Design review of the part built by this model. Coordinates are the model's own, in mm. Face numbers are marked on the shaded views. Give positions to 0.01 mm unless a question says otherwise; leave off trailing zeros. Order: outer loops, then holes, each group sorted by start corner. A loop starts at its lowest first (then second) coordinate and runs counter-clockwise, first axis right, second up.
```python
from build123d import *

# Parameters (mm, degrees)
F0_W        = 40
F0_H        = 30
F0_R        = 2.6
F1_DEPTH    = 6
F2_T1_DEPTH = 31


# Not quite as in the source:
# - a fillet or chamfer that OpenCascade refuses, or shapes differently, is made with other operations: its cross-section is extruded or revolved along the edge and cut away or added


with BuildPart() as f1:
    # F0 (on Top) → F1 (new body)
    with BuildSketch(Plane.XY):
        Rectangle(F0_W, F0_H)
        with Locations((-10, -7)):
            Circle(F0_R, mode=Mode.SUBTRACT)
        with Locations((10, 0)):
            Circle(F0_R, mode=Mode.SUBTRACT)
    extrude(amount=F1_DEPTH)

    # F2: fillet of radius 5 on 4 edges, made by hand

    # F2_s2 → F2_t1 (cut)
    with BuildSketch(Plane.XY.offset(-12.5)):
        with BuildLine():
            add(Edge.make_bspline(
                [(-20, -10), (-20, -15), (-15, -15)],
                knots=[0, 0, 0, 1, 1, 1], degree=2, weights=[1, 1, 1]))
            Line((-15, -15), (-20, -15))
            Line((-20, -15), (-20, -10))
        make_face()
        with BuildLine():
            add(Edge.make_bspline(
                [(15, -15), (20, -15), (20, -10)],
                knots=[0, 0, 0, 1, 1, 1], degree=2, weights=[1, 1, 1]))
            Line((20, -10), (20, -15))
            Line((20, -15), (15, -15))
        make_face()
        with BuildLine():
            add(Edge.make_bspline(
                [(15, 15), (20, 15), (20, 10)],
                knots=[0, 0, 0, 1, 1, 1], degree=2, weights=[1, 1, 1]))
            Line((20, 10), (20, 15))
            Line((20, 15), (15, 15))
        make_face()
        with BuildLine():
            add(Edge.make_bspline(
                [(-15, 15), (-20, 15), (-20, 10)],
                knots=[0, 0, 0, 1, 1, 1], degree=2, weights=[1, 1, 1]))
            Line((-20, 10), (-20, 15))
            Line((-20, 15), (-15, 15))
        make_face()
    extrude(amount=F2_T1_DEPTH, mode=Mode.SUBTRACT)


solid = f1.part
```
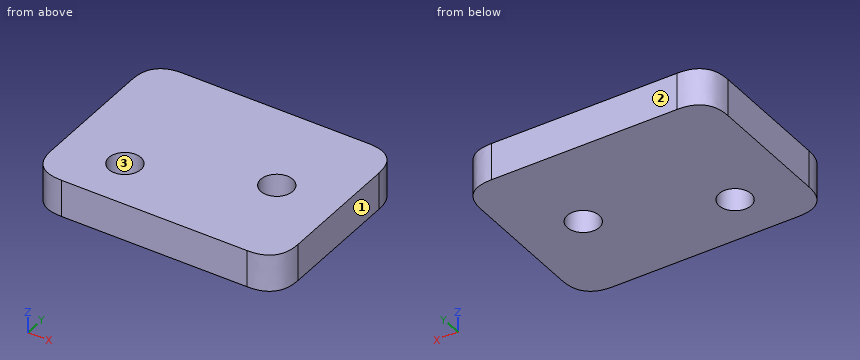
1. Take a section at B-B (y = 0). State the section outline as (x, z) points.
Recorded:
outline: (-20, 0) - (7.4, 0) - (7.4, 6) - (-20, 6) - close; (12.6, 0) - (20, 0) - (20, 6) - (12.6, 6) - close
2. Take a section at C-C (z = 1.75). State how many separate pieces and enclosed holes the cut face has, then the cut area to 3 significant figures.
Recorded:
separate pieces: 1
enclosed holes: 2
area: 1,140 mm2
3. Take a section at A-A (x = -11). State the section outline as (y, z) points.
Recorded:
outline: (-15, 0) - (-9.4, 0) - (-9.4, 6) - (-15, 6) - close; (-4.6, 0) - (15, 0) - (15, 6) - (-4.6, 6) - close
4. Draft analysis for pull direction X (two halves, no side actions). For the marked faces 1, 2 and 3, state which applies: pulls with the +X half, pulls with the -X half, needs draft (parallel to the pull), parting line crosses it, or undercut.
Recorded:
face 1: pulls with the +X half
face 2: needs draft
face 3: undercut
5. For pin 1 (8.5 mm diameter, centred on x = 10, y = 0, fed in from +Z), flat-tipped, find the tip position at first contact; note if it passes through.
Recorded:
pin 1: stops at z = 6
6. For line 1 along Y through (x, z) = (10, 3.35); line 2 along Y through (x, z) = (-10, 2.2); line 3 along X through (y, z) = (0.5, 3), list the stretches that pass through material, from the lowest coordinate up.
Recorded:
line 1: y = -15 to -2.6, 2.6 to 15
line 2: y = -15 to -9.6, -4.4 to 15
line 3: x = -20 to 7.45, 12.55 to 20
